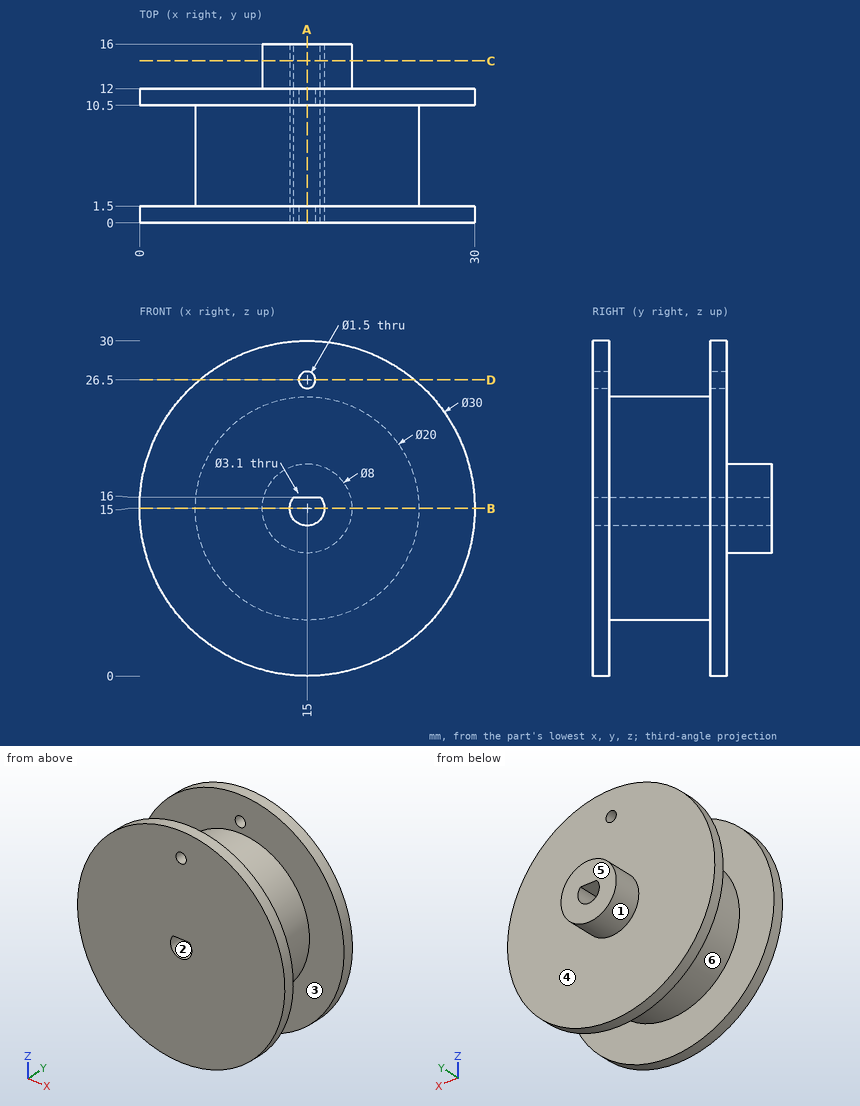
For this review, use the dimensioned drawing (mm, ordinates from the lowest corner) and the shaded views. A direction names the side the tool comes from. Round coordinates to 2 decimals unless told otherwise and drop trailing zeros. Order: outer loops, then holes, each group sorted by start corner. A loop starts at its lowest first (then second) coordinate and runs counter-clockwise, first axis right, second up.
1) Consider section A-A (x = 15). State the section outline as (y, z) points, plus the area to 3 significant figures.
The answers:
outline: (0, 0) - (1.5, 0) - (1.5, 5) - (10.5, 5) - (10.5, 0) - (12, 0) - (12, 11) - (16, 11) - (16, 13.45) - (0, 13.45) - close; (0, 16) - (16, 16) - (16, 19) - (12, 19) - (12, 25.75) - (10.5, 25.75) - (10.5, 25) - (1.5, 25) - (1.5, 25.75) - (0, 25.75) - close; (0, 27.25) - (1.5, 27.25) - (1.5, 30) - (0, 30) - close; (10.5, 27.25) - (12, 27.25) - (12, 30) - (10.5, 30) - close
area: 257 mm2
2) Consider section D-D (z = 26.5). State the section outline as (x, y) points.
The answers:
outline: (5.37, 0) - (14.25, 0) - (14.25, 1.5) - (5.37, 1.5) - close; (5.37, 10.5) - (14.25, 10.5) - (14.25, 12) - (5.37, 12) - close; (15.75, 0) - (24.63, 0) - (24.63, 1.5) - (15.75, 1.5) - close; (15.75, 10.5) - (24.63, 10.5) - (24.63, 12) - (15.75, 12) - close
3) Consider section C-C (y = 14.5). State the section outline as (x, z) points.
The answers:
outline: circle Ø8 at (15, 15); hole (13.82, 16) arc R1.55 ccw (long way) to (16.18, 16) - close
4) Draft analysis for pull direction X (two halves, no side actions). For the marked faces 1, 2 and 3, state which applies: released by +X, released by -X, zero draft, split by the parting line, or undercut.
The answers:
face 1: split by the parting line
face 2: undercut
face 3: zero draft
5) Consider section B-B (z = 15). State the section outline as (x, y) points.
The answers:
outline: (0, 0) - (13.45, 0) - (13.45, 16) - (11, 16) - (11, 12) - (0, 12) - (0, 10.5) - (5, 10.5) - (5, 1.5) - (0, 1.5) - close; (16.55, 0) - (30, 0) - (30, 1.5) - (25, 1.5) - (25, 10.5) - (30, 10.5) - (30, 12) - (19, 12) - (19, 16) - (16.55, 16) - close
6) Machinability: for the marked faces 4, 5 and 6, which of the approach directions +Z, -Z, +X, -X, +Y, -Y give a long, thin tool a straight path to every point of the face, cutting with its end or side? Answer none if there is none.
The answers:
face 4: +Y
face 5: +Z, -Z, +X, -X, +Y
face 6: none
7) For L1, parallel to Y at x = 26, z = 7; L2, parallel to X at y = 6.25, z = 15; L3, parallel to Y at x = 11, z = 8.5, list the stretches that pass through material, from the lowest coordinate up.
The answers:
L1: y = 0 to 1.5, 10.5 to 12
L2: x = 5 to 13.45, 16.55 to 25
L3: y = 0 to 12
8) Clearance check with flat-ended pins moving along their axes: pin 1 Ø3 at (x, y) = (13, 6) entering from +Z; pin 2 Ø10 at (x, z) = (8, 27) entering from +Y; pin 3 Ø2 at (x, z) = (3, 4) entering from -Y; pin 4 Ø5 at (y, z) = (12.5, 21.5) entering from -X. State where each tip first meets the part, or that it passes through.
The answers:
pin 1: stops at z = 24.99
pin 2: stops at y = 12
pin 3: passes through
pin 4: stops at x = 0.56
